from build123d import *
from build123d.topology import SkipClean

# Parameters (mm, degrees)
SKETCH_2_R                = 1.288183927
SKETCH_2_R_2              = 0.75
CUT_EXTRUDE_1_DEPTH       = 13
SKETCH_3_R                = 0.4
CUT_EXTRUDE_2_DEPTH       = 5
SKETCH_8_W                = 0.443463538
SKETCH_8_H                = 2
CUT_EXTRUDE_3_DEPTH       = 7
PATTERN_CIRCULAR_13_COUNT = 12


with BuildPart() as part:
    # Sketch 1 → Revolve 1 (revolve)
    with SkipClean():  # the faces are left unmerged after this step: merging them gives an invalid solid
        with BuildSketch(Plane.XY, mode=Mode.PRIVATE) as revolve_1_sk:
            with BuildLine():
                Line((1, 13.5), (1, 0))
                Line((1, 0), (2, 0))
                Line((2, 0), (2, 14))
                add(Edge.make_bspline(
                    [(1, 13.5), (2, 13.5), (2, 14)],
                    knots=[4.71238898, 4.71238898, 4.71238898, 6.283185307, 6.283185307, 6.283185307], degree=2, weights=[1, 0.707106781, 1]))
            make_face()
            with BuildLine():
                add(Edge.make_bspline(
                    [(1, 14.5), (0, 14.5), (0, 14)],
                    knots=[1.570796327, 1.570796327, 1.570796327, 3.141592654, 3.141592654, 3.141592654], degree=2, weights=[1, 0.707106781, 1]))
                add(Edge.make_bspline(
                    [(0, 14), (0, 13.5), (1, 13.5)],
                    knots=[3.141592654, 3.141592654, 3.141592654, 4.71238898, 4.71238898, 4.71238898], degree=2, weights=[1, 0.707106781, 1]))
                Line((1, 13.5), (1, 14.5))
            make_face()
            with BuildLine():
                Line((1, 14.5), (1, 13.5))
                add(Edge.make_bspline(
                    [(1, 13.5), (2, 13.5), (2, 14)],
                    knots=[4.71238898, 4.71238898, 4.71238898, 6.283185307, 6.283185307, 6.283185307], degree=2, weights=[1, 0.707106781, 1]))
                add(Edge.make_bspline(
                    [(2, 14), (2, 14.5), (1, 14.5)],
                    knots=[0, 0, 0, 1.570796327, 1.570796327, 1.570796327], degree=2, weights=[1, 0.707106781, 1]))
            make_face()
        revolve(revolve_1_sk.sketch.rotate(Axis((1, 20.110661338, 0), (0, -1, 0)), 180), axis=Axis((1, 20.110661338, 0), (0, -1, 0)))
    add(part.part.scale(1), mode=Mode.REPLACE)  # the faces are merged on a copy

    # Sketch 2 → Cut-Extrude 1 (cut)
    with BuildSketch(Plane.XZ):
        with Locations((1, 0)):
            Circle(SKETCH_2_R)
        with Locations((1, 0)):
            Circle(SKETCH_2_R_2, mode=Mode.SUBTRACT)
    extrude(amount=-CUT_EXTRUDE_1_DEPTH, mode=Mode.SUBTRACT)

    # Sketch 3 → Cut-Extrude 2 (cut)
    with BuildSketch(Plane(origin=(0, 0, 0), x_dir=(-1, 0, 0), z_dir=(0, -1, 0))):
        with Locations(Location((-1, 0, 0), (0, 0, 180))):
            Circle(SKETCH_3_R)
    extrude(amount=-CUT_EXTRUDE_2_DEPTH, mode=Mode.SUBTRACT)

    # Sketch 8 → Cut-Revolve 1 (revolve, cut)
    with BuildSketch(Plane.XY):
        with Locations((1.721731769, 10.5)):
            Rectangle(SKETCH_8_W, SKETCH_8_H)
        with Locations((1.721731769, 7.5)):
            Rectangle(SKETCH_8_W, SKETCH_8_H)
    revolve(axis=Axis((1, 0, 0), (0, 1, 0)), mode=Mode.SUBTRACT)

    # Sketch 9 → Cut-Extrude 3 (cut)
    with BuildSketch(Plane(origin=(0, 5.5, 0), x_dir=(-1, 0, 0), z_dir=(0, -1, 0))):
        with BuildLine():
            Line((-1.137321392, 0.737321392), (-1, 0.6))
            Line((-1, 0.6), (-1, 0.75))
            ThreePointArc((-1, 0.75), (-1.068952723, 0.746823622), (-1.137321392, 0.737321392))
        make_face()
        with BuildLine():
            Line((-1, 0.75), (-1, 0.6))
            Line((-1, 0.6), (-0.862678608, 0.737321392))
            ThreePointArc((-0.862678608, 0.737321392), (-0.931047277, 0.746823622), (-1, 0.75))
        make_face()
    cut_extrude_3 = extrude(amount=-CUT_EXTRUDE_3_DEPTH, mode=Mode.SUBTRACT)

    # Pattern Circular 13: Cut-Extrude 3 ×12 about axis
    pattern_circular_13_axis = Axis((1, 0, 0), (0, 1, 0))
    for i in range(1, PATTERN_CIRCULAR_13_COUNT):
        add(cut_extrude_3.rotate(pattern_circular_13_axis, i * 360 / PATTERN_CIRCULAR_13_COUNT), mode=Mode.SUBTRACT)


solid = part.part
CAD build for the part. Positions are in the model's coordinates, mm. A direction names the side the tool comes from. Coordinates: 2 decimals unless noted, no trailing zeros. Loops run counter-clockwise (first coordinate to the right, second up) from the corner with the lowest first, then second, coordinate; pieces in that order, holes last. Notation, with made-up numbers: (-29.5, -31.75) - (-18.5, -31.75) arc R23 cw to (-18.5, -17.75) - close; hole circle Ø8 at (24.25, 73.25). An arc over 180 degrees is marked (long way). Use one line per item in the form item = value. Start each with the question number.
1) Flat gauge pin, fed straight in: pin 1 (0.7 mm diameter, centred on x = 0.5, z = 0, fed in from +Y). Where does the tip first touch, or does it go through?
2) Tool access for faces 1 (the face through (0.6, 7.5, 0.3)), 2 (the face through (1.69, 3.2, -0.29)): list every direction of +Z, -Z, +X, -X, +Y, -Y with a clear straight run to the whole face (end or side of a thin tool).
3) Band-saw the part on A-A (y = 1.75). Give the cut face in (x, z), and give its area (3 significant figures).
4) Two-plate mould, pull along Y, no slides. Class faces 3 (the face through (1.217, 13.507, 0.976)), 4 (the face through (0.6, 10.5, 0.3)): +Y half, -Y half, draft (parallel to the pull), parting line (faces both ways), or undercut.
5) Drill centre lines: L1, parallel to Z at x = 1, y = 3.9; L2, parallel to X at y = 13.75, z = 0.8; L3, parallel to Y at x = 0.6, z = -0.35. Where is each one in solid material? Low to high. Write a range as from..to.
6) Band-saw the part on B-B (y = 10). Give the cut face in (x, z).
Check values:
q1.pin_1 = 14.49
q2.face_1 = none
q2.face_2 = -Y
q3.outline = circle Ø1.5 at (1, 0); hole circle Ø0.8 at (1, 0)
q3.area = 1.26 mm2
q4.face_3 = draft
q4.face_4 = undercut
q5.L1 = -0.75..-0.4, 0.4..0.75
q5.L2 = 0.4..1.6
q5.L3 = 0..6.5, 8.5..9.5, 11.5..14.42
q6.outline = circle Ø1 at (1, 0)
